Could you check a few things on this model? Use its own coordinates, in mm. A direction names the side the tool comes from. Give positions to 0.01 mm unless a question says otherwise; leave off trailing zeros. Put each result on its own line as item: value.
```python
from build123d import *

# Parameters (mm, degrees)
F0_W      = 2.5
F0_H      = 4.3
F1_DEPTH  = 0.01
F4_W      = 3
F4_H      = 2.4
F5_DEPTH  = 2
F0_W_2    = 0.25
F0_H_2    = 26.2
F6_DEPTH  = 0.01
F7_DEPTH  = 0.01
F7_FACE_W = 0.25
F7_FACE_H = 28.7
F6_FACE_W = 0.25
F6_FACE_H = 26.2
F10_R     = 0.2


with BuildPart() as f1:
    # F0 (on Front) → F1 (new body)
    with BuildSketch(Plane.XZ):
        with Locations((1.25, 2.15)):
            Rectangle(F0_W, F0_H)
        Polygon((2.5, 0), (0, 0), (0, -1), (1.02, -1), (1.27, -1), (2.9, -1), (2.9, 0), align=None)
    extrude(amount=F1_DEPTH)

    # F1_face (on face) → F2 (revolve)
    with BuildSketch(Plane(origin=(1.2924908425, -0.01, 1.586996337), x_dir=(1, 0, 0), z_dir=(0, -1, 0))):
        Polygon((-1.2924908425, 2.713003663), (-1.2924908425, -2.586996337), (1.6075091575, -2.586996337), (1.6075091575, -1.586996337), (1.2075091575, -1.586996337), (1.2075091575, 2.713003663), align=None)
    revolve(axis=Axis((0, 0, 1.65), (0, 0, 1)))

    # F4 (on offset) → F5 (cut)
    with BuildSketch(Plane.YZ.offset(2.5)):
        Rectangle(F4_W, F4_H)
    extrude(amount=F5_DEPTH, mode=Mode.SUBTRACT)

    # F0 (on Front) → F6 (join)
    with BuildSketch(Plane.XZ):
        with Locations((1.145, -14.1)):
            Rectangle(F0_W_2, F0_H_2)
    extrude(amount=F6_DEPTH)

    # F0 (on Front) → F7 (join)
    with BuildSketch(Plane.XZ):
        Polygon((-1.02, -29.7), (-1.02, -27.2), (-1.02, -1), (-1.27, -1), (-1.27, -29.7), align=None)
    extrude(amount=F7_DEPTH)

    # F7_face (on face) → F8 (revolve)
    with BuildSketch(Plane(origin=(-1.145, -0.01, -15.35), x_dir=(1, 0, 0), z_dir=(0, -1, 0))):
        Rectangle(F7_FACE_W, F7_FACE_H)
    revolve(axis=Axis((-1.27, 0, -15.35), (0, 0, 1)))

    # F6_face (on face) → F9 (revolve)
    with BuildSketch(Plane(origin=(1.145, -0.01, -14.1), x_dir=(1, 0, 0), z_dir=(0, -1, 0))):
        Rectangle(F6_FACE_W, F6_FACE_H)
    revolve(axis=Axis((1.27, 0, -14.1), (0, 0, -1)))

    # F10
    f10_edges = [f1.edges().sort_by_distance(p)[0] for p in [
        (-2.5, 0.01, 4.3),
    ]]
    fillet(f10_edges, radius=F10_R)


solid = f1.part
```
1. I need wall thicknesses on line 1 (Z direction, x = 1.9, y = 0.1); line 2 (Z direction, x = 0.85, y = 2.55); line 3 (Y direction, x = -2.05, z = 1). Which ranges of each line are inside material? Lowest first, please.
Recorded:
line 1: z = -1 to 4.3
line 2: z = -1 to 0
line 3: y = -1.43 to 1.43
2. For faces 1 (the face through (2.306, -0.967, 2.079)), 2 (the face through (2.5, 0, -0.6)), which set-ups out of +Z, -Z, +X, -X, +Y, -Y let a thin tool reach every point of the face, with its end or its side?
Recorded:
face 1: +Z
face 2: +Z, -Z, +X, +Y, -Y
3. If we section it at A-A (z = -21.5): Count the separate pieces of the cut face and the enclosed holes in it, then the cut area to 3 significant figures.
Recorded:
separate pieces: 2
enclosed holes: 2
area: 0.393 mm^2
4. I'm going to push flat-ended pins straight in: pin 1 (2 mm diameter, centred on y = -0.5, z = -22, fed in from +X); pin 2 (1 mm diameter, centred on x = 1, y = 2, fed in from -Z); pin 3 (3 mm diameter, centred on x = -0.5, y = 1, fed in from -Z). Where does each tip first touch, or does it pass through?
Recorded:
pin 1: stops at x = 1.52
pin 2: stops at z = -1
pin 3: stops at z = -29.7
